```python
from build123d import *

# Parameters (mm, degrees)
SKETCH1_R               = 40
BOSS_EXTRUDE1_DEPTH     = 24
SKETCH2_W               = 80
SKETCH2_H               = 80
SKETCH2_R               = 2
BOSS_EXTRUDE2_DEPTH     = 5
FILLET1_R               = 4
SKETCH3_R               = 34
BOSS_EXTRUDE3_DEPTH     = 100
SKETCH4_R               = 10
BOSS_EXTRUDE4_DEPTH     = 3
SKETCH5_R               = 5
BOSS_EXTRUDE5_DEPTH     = 50
FILLET3_R               = 1
FILLET4_R               = 1
SKETCH6_W               = 26.979088542
SKETCH6_H               = 2
CUT_EXTRUDE1_DEPTH      = 1
CUT_EXTRUDE1_DEPTH_BACK = 81
SKETCH8_R               = 2
BOSS_EXTRUDE6_DEPTH     = 7
FILLET5_R               = 2
SKETCH10_R              = 34
SKETCH10_R_2            = 31.5
CUT_EXTRUDE3_DEPTH      = 15
FILLET6_R               = 2
FILLET7_R               = 2
FILLET8_R               = 2


with BuildPart() as part:
    # Sketch1 → Boss-Extrude1 (new body)
    with BuildSketch(Plane.XY):
        Circle(SKETCH1_R)
    extrude(amount=BOSS_EXTRUDE1_DEPTH)

    # Sketch2 → Boss-Extrude2 (add)
    with BuildSketch(Plane.XY.offset(24)):
        Rectangle(SKETCH2_W, SKETCH2_H)
        with Locations((33, -33)):
            Circle(SKETCH2_R, mode=Mode.SUBTRACT)
        with Locations((-33, 33)):
            Circle(SKETCH2_R, mode=Mode.SUBTRACT)
        with Locations((33, 33)):
            Circle(SKETCH2_R, mode=Mode.SUBTRACT)
        with Locations((-33, -33)):
            Circle(SKETCH2_R, mode=Mode.SUBTRACT)
    extrude(amount=BOSS_EXTRUDE2_DEPTH)

    # Fillet1
    fillet1_edges = [part.edges().sort_by_distance(p)[0] for p in [
        (40, 40, 26.5),
        (-40, 40, 26.5),
        (-40, -40, 26.5),
        (40, -40, 26.5),
    ]]
    fillet(fillet1_edges, radius=FILLET1_R)

    # Sketch3 → Boss-Extrude3 (add)
    with BuildSketch(Plane(origin=(0, 0, 0), x_dir=(-1, 0, 0), z_dir=(0, 0, -1))):
        Circle(SKETCH3_R)
    extrude(amount=BOSS_EXTRUDE3_DEPTH)

    # Sketch4 → Boss-Extrude4 (add)
    with BuildSketch(Plane.XY.offset(29)):
        with Locations((0, -15)):
            Circle(SKETCH4_R)
    extrude(amount=BOSS_EXTRUDE4_DEPTH)

    # Sketch5 → Boss-Extrude5 (add)
    with BuildSketch(Plane.XY.offset(32)):
        with Locations((0, -15)):
            Circle(SKETCH5_R)
    extrude(amount=BOSS_EXTRUDE5_DEPTH)

    # Fillet3
    fillet3_edges = [part.edges().sort_by_distance(p)[0] for p in [
        (-10, -15, 32),
    ]]
    fillet(fillet3_edges, radius=FILLET3_R)

    # Fillet4
    fillet4_edges = [part.edges().sort_by_distance(p)[0] for p in [
        (-5, -15, 82),
    ]]
    fillet(fillet4_edges, radius=FILLET4_R)

    # Sketch6 → Cut-Extrude1 (cut, two sides)
    with BuildSketch(Plane.ZY.offset(40)) as cut_extrude1_sk:
        with Locations((75.489544271, -11)):
            Rectangle(SKETCH6_W, SKETCH6_H)
    extrude(amount=CUT_EXTRUDE1_DEPTH, mode=Mode.SUBTRACT)
    extrude(cut_extrude1_sk.sketch, amount=-CUT_EXTRUDE1_DEPTH_BACK, mode=Mode.SUBTRACT)

    # Sketch8 → Boss-Extrude6 (add)
    with BuildSketch(Plane.XY.offset(29)):
        with BuildLine():
            Line((-36, -24), (-40, -24))
            Line((-40, -24), (-40, -36))
            ThreePointArc((-40, -36), (-38.828427125, -38.828427125), (-36, -40))
            Line((-36, -40), (-29, -40))
            Line((-29, -40), (-29, -32))
            Line((-29, -32), (-36, -24))
        make_face()
        with Locations((-33, -33)):
            Circle(SKETCH8_R, mode=Mode.SUBTRACT)
        with BuildLine():
            Line((29, -32), (29, -40))
            Line((29, -40), (36, -40))
            ThreePointArc((36, -40), (38.828427125, -38.828427125), (40, -36))
            Line((40, -36), (40, -24))
            Line((40, -24), (36, -24))
            Line((36, -24), (29, -32))
        make_face()
        with Locations((33, -33)):
            Circle(SKETCH8_R, mode=Mode.SUBTRACT)
        with BuildLine():
            Line((-40, 36), (-40, 24))
            Line((-40, 24), (-36, 24))
            Line((-36, 24), (-29, 32))
            Line((-29, 32), (-29, 40))
            Line((-29, 40), (-36, 40))
            ThreePointArc((-36, 40), (-38.828427125, 38.828427125), (-40, 36))
        make_face()
        with Locations((-33, 33)):
            Circle(SKETCH8_R, mode=Mode.SUBTRACT)
        with BuildLine():
            Line((36, 40), (29, 40))
            Line((29, 40), (29, 32))
            Line((29, 32), (36, 24))
            Line((36, 24), (40, 24))
            Line((40, 24), (40, 36))
            ThreePointArc((40, 36), (38.828427125, 38.828427125), (36, 40))
        make_face()
        with Locations((33, 33)):
            Circle(SKETCH8_R, mode=Mode.SUBTRACT)
    extrude(amount=BOSS_EXTRUDE6_DEPTH)

    # Fillet5
    fillet5_edges = [part.edges().sort_by_distance(p)[0] for p in [
        (-36, -24, 32.5),
        (-40, -24, 32.5),
        (-29, -40, 32.5),
        (-29, -32, 32.5),
        (36, -24, 32.5),
        (29, -32, 32.5),
        (29, -40, 32.5),
        (40, -24, 32.5),
        (-36, 24, 32.5),
        (-29, 32, 32.5),
        (-29, 40, 32.5),
        (-40, 24, 32.5),
        (36, 24, 32.5),
        (40, 24, 32.5),
        (29, 40, 32.5),
        (29, 32, 32.5),
    ]]
    fillet(fillet5_edges, radius=FILLET5_R)

    # Sketch10 → Cut-Extrude3 (cut)
    with BuildSketch(Plane(origin=(0, 0, -100), x_dir=(-1, 0, 0), z_dir=(0, 0, -1))):
        Circle(SKETCH10_R)
        Circle(SKETCH10_R_2, mode=Mode.SUBTRACT)
    extrude(amount=-CUT_EXTRUDE3_DEPTH, mode=Mode.SUBTRACT)

    # Fillet6
    fillet6_edges = [part.edges().sort_by_distance(p)[0] for p in [
        (31.5, 0, -100),
    ]]
    fillet(fillet6_edges, radius=FILLET6_R)

    # Fillet7
    fillet7_edges = [part.edges().sort_by_distance(p)[0] for p in [
        (34, 0, -85),
    ]]
    fillet(fillet7_edges, radius=FILLET7_R)

    # Fillet8
    fillet8_edges = [part.edges().sort_by_distance(p)[0] for p in [
        (-40, 0, 0),
    ]]
    fillet(fillet8_edges, radius=FILLET8_R)


solid = part.part
```
The model under review builds one solid part; all positions refer to its coordinate system, in mm. A direction names the side the tool comes from. Round coordinates to 2 decimals unless told otherwise and drop trailing zeros. Write each loop counter-clockwise with the first axis right and the second up, starting at its lowest first coordinate (ties: lowest second). Pieces come first, ordered by that corner, then holes.
(1) Mouldability with a two-part tool opening along X and no side actions: class faces 4 (the cylindrical face through (33.923, 31.226, 29.916)), 5 (the flat face through (40, -1, 27)), 6 (the flat face through (30, -30, 24)), 7 (the cylindrical face through (33.923, -34.774, 29.916)) as +X half, -X half, draft (parallel to the pull), parting line (faces both ways), or undercut.
(2) We need section A-A on z = 58. Give the boundary of the cut face in (x, y).
(3) Machinability: for faces 1 (the flat face through (30, 30, 24)), 2 (the cylindrical face through (-1.08, -19.88, 56.16)), 3 (the flat face through (-30, 30, 24)), which of the approach directions +Z, -Z, +X, -X, +Y, -Y give a long, thin tool a straight path to every point of the face, cutting with its end or side? Answer none if there is none.
(4) Wall thickness on L1, parallel to X at y = 27.5, z = 15.5; L2, parallel to Z at x = -9.5, y = 2; L3, parallel to Y at x = -33, z = 29.5: over which ranges is each line inside the solid? List them lowest first.
(5) We need section B-B on z = -18.5. Give the boundary of the cut face in (x, y).
(6) Insertion check: pin 1 (12 mm diameter, centred on x = 16, y = -14, fed in from +Z); pin 2 (0.9 mm diameter, centred on x = -37.5, z = 32.5, fed in from +Y); pin 3 (6 mm diameter, centred on x = -25, z = -50, fed in from +Y). Each pin has a flat end and moves straight along its axis. Give the tip position at first contact, or say it passes through.
Findings below:
1. face 4: undercut
1. face 5: +X half
1. face 6: draft
1. face 7: undercut
2. outline: circle Ø10 at (0, -15)
3. face 1: -Z, +X, +Y
3. face 2: +Z
3. face 3: -Z, -X, +Y
4. L1: x = -29.05 to 29.05
4. L2: z = -100 to 29
4. L3: y = -40 to -35, -31 to -27.43, 27.43 to 31, 35 to 40
5. outline: circle Ø68 at (0, 0)
6. pin 1: stops at z = 29
6. pin 2: stops at y = 39.86
6. pin 3: stops at y = 25.92
